Part model, mm, in its own coordinate system. Face numbers are marked on the shaded views. A direction names the side the tool comes from. Give positions to 0.01 mm unless a question says otherwise; leave off trailing zeros. Order: outer loops, then holes, each group sorted by start corner. A loop starts at its lowest first (then second) coordinate and runs counter-clockwise, first axis right, second up. Notation, with made-up numbers: (-29, 16.25) - (10, 16.25) arc R25 cw to (10, 34.25) - close; hole circle Ø4 at (76.25, -39). An arc over 180 degrees is marked (long way). Use one line per item in the form item = value. Start each with the question number.
1. Pull direction X, two halves, no side cores. Call the marked faces 3, 4, 5 and 6: +X half, -X half, draft (parallel to the pull), parting line (faces both ways), or undercut.
2. Pin check, flat tips, straight feed: P1, Ø5, axis at x = 30.5, z = 0, coming from the +Y side; P2, Ø3, axis at x = 8, z = 0, coming from the +Y side; P3, Ø1.1, axis at x = -18, y = 0.5, coming from the -Z side; P4, Ø0.8, axis at y = 0.5, z = 3.5, coming from the +X side. Stop position of each tip, or through.
3. Band-saw the part on C-C, the plane z = 1. List the corners of the cut face in (x, y), plus the area to 3 significant figures.
4. Band-saw the part on A-A, the plane x = 0. List the corners of the cut face in (y, z).
5. Drill centre lines: line 1 (X direction, y = 7.75, z = 0); line 2 (X direction, y = 6.75, z = 0); line 3 (X direction, y = 19.75, z = -1.5). Where is each one in solid material? Low to high.
6. Band-saw the part on B-B, the plane y = 4. List the corners of the cut face in (x, z).
7. Band-saw the part on D-D, the plane x = 30.5. List the corners of the cut face in (y, z), plus the area to 3 significant figures.
8. Tool access for the marked faces 1 and 2: list every direction of +Z, -Z, +X, -X, +Y, -Y with a clear straight run to the whole face (end or side of a thin tool).
from build123d import *

# Parameters (mm, degrees)
CROQUIS1_W              = 85
CROQUIS1_H              = 15
SALIENTE_EXTRUIR1_DEPTH = 25
CROQUIS2_R              = 5.35
CORTAR_EXTRUIR1_DEPTH   = 50.874843358
CROQUIS3_R              = 4.15
CORTAR_EXTRUIR2_DEPTH   = 18
REDONDEO1_R             = 2
CROQUIS6_R              = 1.75
CORTAR_EXTRUIR4_DEPTH   = 50.874843358
CORTAR_EXTRUIR7_DEPTH   = 1


with BuildPart() as part:
    # Croquis1 → Saliente-Extruir1 (new body)
    with BuildSketch(Plane(origin=(0, 0, 0), x_dir=(1, 0, 0), z_dir=(0, 1, 0))):
        Rectangle(CROQUIS1_W, CROQUIS1_H)
    extrude(amount=SALIENTE_EXTRUIR1_DEPTH)

    # Croquis2 → Cortar-Extruir1 (cut, through all)
    with BuildSketch(Plane(origin=(0, 0, 0), x_dir=(-1, 0, 0), z_dir=(0, -1, 0))):
        with Locations(Location((0, 0, 0), (0, 0, 90))):
            Circle(CROQUIS2_R)
    extrude(amount=-CORTAR_EXTRUIR1_DEPTH, mode=Mode.SUBTRACT)

    # Croquis3 → Cortar-Extruir2 (cut)
    with BuildSketch(Plane(origin=(0, 25, 0), x_dir=(1, 0, 0), z_dir=(0, 1, 0))):
        with Locations(Location((-30.5, 0, 0), (0, 0, 270))):
            Circle(CROQUIS3_R)
        with Locations(Location((30.5, 0, 0), (0, 0, 270))):
            Circle(CROQUIS3_R)
    extrude(amount=-CORTAR_EXTRUIR2_DEPTH, mode=Mode.SUBTRACT)

    # Redondeo1
    redondeo1_edges = [part.edges().sort_by_distance(p)[0] for p in [
        (0, 0, 7.5),
        (-42.5, 0, 0),
        (0, 0, -7.5),
        (42.5, 0, 0),
        (42.5, 12.5, 7.5),
        (-42.5, 12.5, 7.5),
        (-42.5, 12.5, -7.5),
        (42.5, 12.5, -7.5),
    ]]
    fillet(redondeo1_edges, radius=REDONDEO1_R)

    # Croquis6 → Cortar-Extruir4 (cut, through all)
    with BuildSketch(Plane(origin=(0, 25, 0), x_dir=(1, 0, 0), z_dir=(0, 1, 0))):
        with Locations(Location((8, 0, 0), (0, 0, 270))):
            Circle(CROQUIS6_R)
        with Locations(Location((-8, 0, 0), (0, 0, 270))):
            Circle(CROQUIS6_R)
    extrude(amount=-CORTAR_EXTRUIR4_DEPTH, mode=Mode.SUBTRACT)

    # Croquis7 → Cortar-Extruir7 (cut)
    # profile 1 of 2: a face of its own
    with BuildSketch(Plane.XZ):
        Polygon((-15.735816649, 3.627604167), (-15.735816649, 2.333333333), (-22.735816649, 2.333333333), (-22.735816649, 2.961538462), (-16.453765367, 2.961538462), (-16.453765367, 4.038461538), align=None)
    # profile 2 of 2: a face of its own
    with BuildSketch(Plane.XZ):
        with BuildLine():
            add(Edge.make_bspline(
                [(-19.238621136, -0.269230769), (-19.126426361, -0.269886806), (-18.908486392, -0.271161165), (-18.590917108, -0.285338008), (-18.292996529, -0.308888691), (-18.014710402, -0.341163442), (-17.755986857, -0.380439385), (-17.517517395, -0.432870416), (-17.298198005, -0.492495828), (-17.097314503, -0.56160137), (-16.912157049, -0.639574708), (-16.739313868, -0.724451126), (-16.579004397, -0.819552716), (-16.428820359, -0.919606638), (-16.290437881, -1.02826913), (-16.164119024, -1.144394069), (-16.049787516, -1.269133369), (-15.946082617, -1.40001997), (-15.85574243, -1.537881039), (-15.774339916, -1.678466778), (-15.707527896, -1.824257937), (-15.652629856, -1.973924855), (-15.608641448, -2.127032284), (-15.578179561, -2.284212853), (-15.559088147, -2.445504533), (-15.557257753, -2.554366181), (-15.556329469, -2.609575321)],
                knots=[0, 0, 0, 0, 1.646377244, 3.198111528, 4.663803227, 6.031090796, 7.308794487, 8.502186765, 9.612154809, 10.642545331, 11.617106989, 12.558866172, 13.465886467, 14.35053239, 15.20542558, 16.045215227, 16.865619885, 17.686225247, 18.492864914, 19.282407821, 20.068097601, 20.842842034, 21.620163247, 22.403093475, 23.190129512, 24, 24, 24, 24], degree=3))
            add(Edge.make_bspline(
                [(-15.556329469, -2.609575321), (-15.5573051, -2.665246277), (-15.559245322, -2.775958295), (-15.577893207, -2.939639046), (-15.608835453, -3.099538409), (-15.652677402, -3.254974687), (-15.707068755, -3.40722466), (-15.77524299, -3.555097475), (-15.854600724, -3.699511638), (-15.947848479, -3.838172213), (-16.051813031, -3.972601444), (-16.169338369, -4.09949737), (-16.299237807, -4.218871542), (-16.440121535, -4.332222152), (-16.594691705, -4.436333347), (-16.760259925, -4.535480211), (-16.939721654, -4.624224283), (-17.13008259, -4.709693633), (-17.336609907, -4.783467607), (-17.558139428, -4.850000097), (-17.797287802, -4.903758035), (-18.052800293, -4.948536579), (-18.325615259, -4.983226371), (-18.61514789, -5.008491655), (-18.921588672, -5.021837825), (-19.13110437, -5.024351228), (-19.238621136, -5.025641026)],
                knots=[0, 0, 0, 0, 0.810914788, 1.612654377, 2.396697861, 3.181598691, 3.963628158, 4.749916497, 5.551656086, 6.361998678, 7.18212741, 8.025565596, 8.878627764, 9.750805457, 10.657531673, 11.591944965, 12.560506719, 13.57287815, 14.630710178, 15.753379473, 16.941251878, 18.199788006, 19.531962791, 20.947069417, 22.433333509, 24, 24, 24, 24], degree=3))
            add(Edge.make_bspline(
                [(-19.238621136, -5.025641026), (-19.345668552, -5.024336246), (-19.554246076, -5.021793936), (-19.859313556, -5.008658775), (-20.147290215, -4.982663334), (-20.41897767, -4.950511076), (-20.672762824, -4.904710628), (-20.911058869, -4.85264359), (-21.131809347, -4.787929851), (-21.337247456, -4.71516142), (-21.526675746, -4.631546669), (-21.704586114, -4.542018264), (-21.870019237, -4.443479984), (-22.024587159, -4.338747894), (-22.166692715, -4.226360749), (-22.296687112, -4.106481098), (-22.414484608, -3.979017693), (-22.519869643, -3.844284532), (-22.612031928, -3.703442631), (-22.694410187, -3.559510505), (-22.761255036, -3.409615396), (-22.817693438, -3.257088604), (-22.861636248, -3.100490939), (-22.891723593, -2.939976001), (-22.912883478, -2.776069471), (-22.914494251, -2.665265538), (-22.915303828, -2.609575321)],
                knots=[0, 0, 0, 0, 1.56130642, 3.042141888, 4.451772327, 5.777565838, 7.030558081, 8.211376819, 9.333164717, 10.383253789, 11.387583522, 12.350962576, 13.286244149, 14.193812918, 15.072134482, 15.925989337, 16.770211267, 17.600669898, 18.417446232, 19.22325363, 20.01647746, 20.807971184, 21.593601364, 22.38506573, 23.188331689, 24, 24, 24, 24], degree=3))
            add(Edge.make_bspline(
                [(-22.915303828, -2.609575321), (-22.914366612, -2.554368424), (-22.912518605, -2.445511199), (-22.893556216, -2.284187121), (-22.86263495, -2.127251692), (-22.820644024, -1.974391185), (-22.767276046, -1.825292768), (-22.699393956, -1.681417008), (-22.620661292, -1.5408638), (-22.531088152, -1.404274494), (-22.428439667, -1.274252399), (-22.314913491, -1.150052566), (-22.187662157, -1.034810992), (-22.048722516, -0.927510387), (-21.899273474, -0.825687939), (-21.737842843, -0.731518276), (-21.563380224, -0.646807414), (-21.377200643, -0.567086628), (-21.174840747, -0.496812905), (-20.954351598, -0.435206972), (-20.7145135, -0.383849808), (-20.456038463, -0.342548111), (-20.178733027, -0.308499017), (-19.882108942, -0.285449523), (-19.566422129, -0.271149875), (-19.349882069, -0.269882145), (-19.238621136, -0.269230769)],
                knots=[0, 0, 0, 0, 0.810940842, 1.599017053, 2.38298203, 3.159479784, 3.926441347, 4.70693857, 5.494146311, 6.292334103, 7.104379492, 7.925868426, 8.762126819, 9.623561095, 10.503686106, 11.41783325, 12.366995289, 13.351843594, 14.392337808, 15.512229747, 16.713911458, 17.994391108, 19.357476964, 20.818259213, 22.365182633, 24, 24, 24, 24], degree=3))
        make_face()
        with BuildLine():
            add(Edge.make_bspline(
                [(-19.235816649, -0.897435897), (-19.329314047, -0.897674792), (-19.510774136, -0.898138438), (-19.774460658, -0.91025084), (-20.020401317, -0.926751302), (-20.248908385, -0.948033902), (-20.459208427, -0.97963978), (-20.652747737, -1.015053418), (-20.828502395, -1.058149393), (-20.987677411, -1.109140103), (-21.132977611, -1.167215999), (-21.268172835, -1.230635754), (-21.394902211, -1.298728786), (-21.511878588, -1.375068296), (-21.620266383, -1.457922738), (-21.719754119, -1.547428165), (-21.809907706, -1.643427165), (-21.916883678, -1.77632125), (-22.028736694, -1.950902188), (-22.124938828, -2.171995858), (-22.185786987, -2.39927863), (-22.19350354, -2.553588256), (-22.197355111, -2.630608974)],
                knots=[0, 0, 0, 0, 1.459116078, 2.831857795, 4.118796693, 5.306371758, 6.412361096, 7.436813035, 8.376339383, 9.234574298, 10.043323891, 10.816788787, 11.564361537, 12.286735248, 12.994408768, 13.691741332, 14.372975427, 15.047457468, 16.352811911, 17.594285292, 18.799233213, 20, 20, 20, 20], degree=3))
            add(Edge.make_bspline(
                [(-22.197355111, -2.630608974), (-22.194159549, -2.708124318), (-22.187775023, -2.862994964), (-22.126177549, -3.089262554), (-22.03323847, -3.308923094), (-21.923343459, -3.481066975), (-21.8186868, -3.612032062), (-21.729457503, -3.705866042), (-21.629545769, -3.791990139), (-21.521747177, -3.873674289), (-21.404002208, -3.94859244), (-21.276877058, -4.016718716), (-21.140018702, -4.078885411), (-21.044479224, -4.114303503), (-20.995632354, -4.132411859)],
                knots=[0, 0, 0, 0, 1.353760809, 2.704726607, 4.075137775, 5.516104923, 6.260822281, 7.007110065, 7.778089737, 8.566572457, 9.372053459, 10.217411131, 11.088608312, 12, 12, 12, 12], degree=3))
            add(Edge.make_bspline(
                [(-20.995632354, -4.132411859), (-20.933172875, -4.153515395), (-20.806353347, -4.196364622), (-20.609626043, -4.251588171), (-20.403220515, -4.295078969), (-20.188370281, -4.334205701), (-19.963490879, -4.360911812), (-19.729278111, -4.382407439), (-19.485555387, -4.395068813), (-19.319965404, -4.396638315), (-19.235816649, -4.397435897)],
                knots=[0, 0, 0, 0, 0.884706709, 1.796334032, 2.740027952, 3.714592787, 4.726048262, 5.777819803, 6.87074269, 8, 8, 8, 8], degree=3))
            add(Edge.make_bspline(
                [(-19.235816649, -4.397435897), (-19.151669702, -4.396556249), (-18.987039924, -4.394835257), (-18.746186408, -4.383528181), (-18.517027725, -4.365358649), (-18.299355986, -4.340766586), (-18.093558624, -4.307006884), (-17.899341146, -4.266464843), (-17.716755909, -4.218933951), (-17.545332043, -4.164414601), (-17.38568569, -4.102972048), (-17.237469269, -4.03509645), (-17.099897025, -3.962663991), (-16.973363843, -3.883976736), (-16.857298581, -3.799986068), (-16.754029437, -3.708470792), (-16.660355489, -3.613062092), (-16.553430354, -3.479427706), (-16.444406962, -3.304479133), (-16.344075443, -3.086787836), (-16.286458857, -2.860246548), (-16.278335483, -2.70709964), (-16.274278187, -2.630608974)],
                knots=[0, 0, 0, 0, 1.313668642, 2.570134578, 3.763346207, 4.902004944, 5.98888779, 7.017888835, 7.998425394, 8.933058446, 9.82474457, 10.667209444, 11.476765193, 12.250262638, 12.991704352, 13.7104269, 14.401925311, 15.076585796, 16.378385137, 17.609787933, 18.806186071, 20, 20, 20, 20], degree=3))
            add(Edge.make_bspline(
                [(-16.274278187, -2.630608974), (-16.278335846, -2.553184539), (-16.286458556, -2.39819462), (-16.343924357, -2.169347957), (-16.443472852, -1.950105943), (-16.554134391, -1.776560965), (-16.658462613, -1.643095185), (-16.749186831, -1.54884971), (-16.848975533, -1.460740005), (-16.956904441, -1.377816535), (-17.073939817, -1.301550513), (-17.200650763, -1.233429615), (-17.335858551, -1.170046263), (-17.481125692, -1.111845682), (-17.640540674, -1.061327523), (-17.815408316, -1.016173608), (-18.0091284, -0.980781455), (-18.220016384, -0.949896763), (-18.44880436, -0.926348938), (-18.695312028, -0.910293198), (-18.959454547, -0.898116523), (-19.141850896, -0.897667316), (-19.235816649, -0.897435897)],
                knots=[0, 0, 0, 0, 1.207964612, 2.418129846, 3.655795183, 4.951004962, 5.620895151, 6.296795572, 6.989224116, 7.696855977, 8.419187164, 9.166715907, 9.940135271, 10.748837255, 11.607021648, 12.548275234, 13.5654991, 14.678641405, 15.874140913, 17.15372626, 18.533675393, 20, 20, 20, 20], degree=3))
        make_face(mode=Mode.SUBTRACT)
    extrude(amount=-CORTAR_EXTRUIR7_DEPTH, mode=Mode.SUBTRACT)


solid = part.part
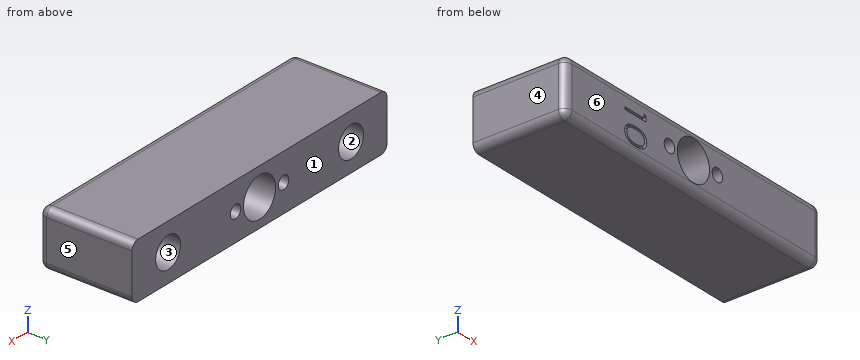
From the geometry:
q1.face_3 = undercut
q1.face_4 = -X half
q1.face_5 = +X half
q1.face_6 = draft
q2.P1 = 7
q2.P2 = through
q2.P3 = -7.26
q2.P4 = 42.17
q3.outline = (-42.5, 2) arc R2 ccw to (-40.5, 0) - (-9.44, 0) - (-9.44, 25) - (-26.47, 25) - (-26.47, 7) - (-34.53, 7) - (-34.53, 25) - (-42.5, 25) - close; (-6.56, 0) - (-5.26, 0) - (-5.26, 25) - (-6.56, 25) - close; (5.26, 0) - (6.56, 0) - (6.56, 25) - (5.26, 25) - close; (9.44, 0) - (40.5, 0) arc R2 ccw to (42.5, 2) - (42.5, 25) - (34.53, 25) - (34.53, 7) - (26.47, 7) - (26.47, 25) - (9.44, 25) - close
q3.area = 1,430 mm²
q4.outline = (0, -5.5) arc R2 ccw to (2, -7.5) - (25, -7.5) - (25, -5.35) - (0, -5.35) - close; (0, 5.35) - (25, 5.35) - (25, 7.5) - (2, 7.5) arc R2 ccw to (0, 5.5) - close
q5.line_1 = -42.5 to -34.65, -26.35 to -9.75, -6.25 to -5.35, 5.35 to 6.25, 9.75 to 26.35, 34.65 to 42.5
q5.line_2 = -42.5 to -9.75, -6.25 to -5.35, 5.35 to 6.25, 9.75 to 42.5
q5.line_3 = -42.5 to -34.37, -26.63 to -8.9, -7.1 to -5.14, 5.14 to 7.1, 8.9 to 26.63, 34.37 to 42.5
q6.outline = (-42.5, -5.5) arc R2 ccw to (-40.5, -7.5) - (40.5, -7.5) arc R2 ccw to (42.5, -5.5) - (42.5, 5.5) arc R2 ccw to (40.5, 7.5) - (-40.5, 7.5) arc R2 ccw to (-42.5, 5.5) - close; hole circle Ø3.5 at (-8, 0); hole circle Ø10.7 at (0, 0); hole circle Ø3.5 at (8, 0)
q7.outline = (0, -5.5) arc R2 ccw to (2, -7.5) - (25, -7.5) - (25, -4.15) - (7, -4.15) - (7, 4.15) - (25, 4.15) - (25, 7.5) - (2, 7.5) arc R2 ccw to (0, 5.5) - close
q7.area = 224 mm²
q8.face_1 = +Z, -Z, +X, -X, +Y
q8.face_2 = +Y
